```python
from build123d import *

# Parameters (mm, degrees)
SKETCH1_R           = 1.6
BOSS_EXTRUDE2_DEPTH = 2
BOSS_EXTRUDE3_DEPTH = 25
CUT_EXTRUDE1_REACH  = 92.161


with BuildPart() as part:
    # Sketch1 → Boss-Extrude2 (new body)
    with BuildSketch(Plane(origin=(0, 0, 0), x_dir=(1, 0, 0), z_dir=(0, 1, 0))):
        with BuildLine():
            Line((5, 0), (65, 0))
            ThreePointArc((65, 0), (68.535533906, -1.464466094), (70, -5))
            Line((70, -5), (70, -45))
            ThreePointArc((70, -45), (68.535533906, -48.535533906), (65, -50))
            Line((65, -50), (5, -50))
            ThreePointArc((5, -50), (1.464466094, -48.535533906), (0, -45))
            Line((0, -45), (0, -5))
            ThreePointArc((0, -5), (1.464466094, -1.464466094), (5, 0))
        make_face()
        with Locations(Location((6.4, -6.1, 0), (0, 0, 270))):
            Circle(SKETCH1_R, mode=Mode.SUBTRACT)
        with Locations(Location((63.6, -6.1, 0), (0, 0, 270))):
            Circle(SKETCH1_R, mode=Mode.SUBTRACT)
        with Locations(Location((6.4, -43.9, 0), (0, 0, 270))):
            Circle(SKETCH1_R, mode=Mode.SUBTRACT)
        with Locations(Location((63.6, -43.9, 0), (0, 0, 270))):
            Circle(SKETCH1_R, mode=Mode.SUBTRACT)
    extrude(amount=BOSS_EXTRUDE2_DEPTH)

    # Sketch2 → Boss-Extrude3 (add)
    with BuildSketch(Plane(origin=(0, 2, 0), x_dir=(1, 0, 0), z_dir=(0, 1, 0))):
        with BuildLine():
            Line((5, 0), (65, 0))
            ThreePointArc((65, 0), (68.535533906, -1.464466094), (70, -5))
            Line((70, -5), (70, -45))
            ThreePointArc((70, -45), (68.535533906, -48.535533906), (65, -50))
            Line((65, -50), (5, -50))
            ThreePointArc((5, -50), (1.464466094, -48.535533906), (0, -45))
            Line((0, -45), (0, -5))
            ThreePointArc((0, -5), (1.464466094, -1.464466094), (5, 0))
        make_face()
        with BuildLine():
            Line((2, -5), (2, -45))
            ThreePointArc((2, -45), (2.878679656, -47.121320344), (5, -48))
            Line((5, -48), (65, -48))
            ThreePointArc((65, -48), (67.121320344, -47.121320344), (68, -45))
            Line((68, -45), (68, -5))
            ThreePointArc((68, -5), (67.121320344, -2.878679656), (65, -2))
            Line((65, -2), (5, -2))
            ThreePointArc((5, -2), (2.878679656, -2.878679656), (2, -5))
        make_face(mode=Mode.SUBTRACT)
    extrude(amount=BOSS_EXTRUDE3_DEPTH)

    # Sketch3 → Cut-Extrude1 (cut, up to next)
    with BuildSketch(Plane(origin=(0, 0, 0), x_dir=(-1, 0, 0), z_dir=(0, 0, -1)), mode=Mode.PRIVATE) as cut_extrude1_sk1:
        with BuildLine():
            Line((-13.428689643, 24), (-18.428689643, 24))
            ThreePointArc((-18.428689643, 24), (-19.842903206, 23.414213562), (-20.428689643, 22))
            Line((-20.428689643, 22), (-20.428689643, 20))
            ThreePointArc((-20.428689643, 20), (-19.842903206, 18.585786438), (-18.428689643, 18))
            Line((-18.428689643, 18), (-13.428689643, 18))
            ThreePointArc((-13.428689643, 18), (-12.014476081, 18.585786438), (-11.428689643, 20))
            Line((-11.428689643, 20), (-11.428689643, 22))
            ThreePointArc((-11.428689643, 22), (-12.014476081, 23.414213562), (-13.428689643, 24))
        make_face()
    cut_extrude1_tool1 = extrude(cut_extrude1_sk1.sketch, amount=-CUT_EXTRUDE1_REACH, mode=Mode.PRIVATE) & part.part
    add(cut_extrude1_tool1.solids().sort_by_distance((15.92869, 21, 0))[0], mode=Mode.SUBTRACT)


solid = part.part
```
Here's how the part is built. I have some questions about the finished solid (model axes, mm). A direction names the side the tool comes from. Round coordinates to 2 decimals unless told otherwise and drop trailing zeros. Write each loop counter-clockwise with the first axis right and the second up, starting at its lowest first coordinate (ties: lowest second). Pieces come first, ordered by that corner, then holes. Notation, with made-up numbers: M 70,86 L 108,86 A20 ccw 108,115 Z; hole C 45,23 d7. An arc over 180 degrees is marked long. Answer as CSV lines item,"result". Start each with the question number.
1. Suppose I cut it at D-D on x = 25.5. Write out the boundary of the cut face in (y, z), then the cut area to 3 significant figures.
2. On a 3-axis mill with a long thin cutter (end or side, diameter ignored), from which of +Z, -Z, +X, -X, +Y, -Y can I reach the whole of each face in a straight line? I mean faces 1 (the flat face through (35, 14, 2)), 2 (the flat face through (0, 13, 25)), 3 (the cylindrical face through (19.858, 18.601, 0.986)). Say none if no direction works.
3. Suppose I cut it at B-B on z = 6.1. Write out the boundary of the cut face in (x, y).
4. I'm going to push flat-ended pins straight in: pin 1 Ø4 at (x, z) = (6.4, 43.9) entering from +Y; pin 2 Ø0.6 at (y, z) = (21, 1.5) entering from +X; pin 3 Ø1.6 at (y, z) = (21.5, 1) entering from -X. Where does each tip first touch, or does it pass through?
5. I need wall thicknesses on probe 1 along X at (y, z) = (0.95, 43.9); probe 2 along X at (y, z) = (18, 9); probe 3 along Z at (x, y) = (17, 25). Which ranges of each line are inside material? Lowest first, please.
6. Suppose I cut it at C-C on y = 8.25. Write out the boundary of the cut face in (x, z).
7. Thinking about a two-plate mould opening in Y: for faces 4 (the flat face through (11.429, 21, 1)), 5 (the flat face through (35, 13, 50)), 6 (the flat face through (35, 0, 25)), 7 (the flat face through (35, 27, 1)), which applies, released by +Y, released by -Y, zero draft, split by the parting line, or undercut?
8. Suppose I cut it at A-A on x = 63.6. Write out the boundary of the cut face in (y, z).
Check result:
1,outline,"M 0,0 L 27,0 L 27,2 L 2,2 L 2,48 L 27,48 L 27,50 L 0,50 Z"
1,area,"200 mm2"
2,face 1,"+Y"
2,face 2,"+Z, -Z, -X, +Y, -Y"
2,face 3,"-Z"
3,outline,"M 0,0 L 4.8,0 L 4.8,2 L 2,2 L 2,27 L 0,27 Z; M 8,0 L 62,0 L 62,2 L 8,2 Z; M 65.2,0 L 70,0 L 70,27 L 68,27 L 68,2 L 65.2,2 Z"
4,pin 1,"stops at y = 2"
4,pin 2,"stops at x = 68.84"
4,pin 3,"stops at x = 1.16"
5,probe 1,"x = 0 to 4.8, 8 to 62, 65.2 to 70"
5,probe 2,"x = 0 to 2, 68 to 70"
5,probe 3,"z = 0 to 2, 48 to 50"
6,outline,"M 0,5 A5 ccw 5,0 L 65,0 A5 ccw 70,5 L 70,45 A5 ccw 65,50 L 5,50 A5 ccw 0,45 Z; hole M 2,5 A3 ccw 5,2 L 65,2 A3 ccw 68,5 L 68,45 A3 ccw 65,48 L 5,48 A3 ccw 2,45 Z"
7,face 4,"undercut"
7,face 5,"zero draft"
7,face 6,"released by -Y"
7,face 7,"released by +Y"
8,outline,"M 0,0 L 27,0 L 27,2 L 2,2 L 2,4.5 L 0,4.5 Z; M 0,7.7 L 2,7.7 L 2,42.3 L 0,42.3 Z; M 0,45.5 L 2,45.5 L 2,48 L 27,48 L 27,50 L 0,50 Z"
